Autodesk Inventor part; units mm, degrees
ref_plane "YZ Plane" through (0, 0, 0) normal (1, 0, 0) x (0, 1, 0)
ref_plane "XZ Plane" through (0, 0, 0) normal (0, 1, 0) x (-1, 0, 0)
ref_plane "XY Plane" through (0, 0, 0) normal (0, 0, 1) x (1, 0, 0)
sketch "Sketch2" plane through (0, 0, 0) normal (0, 0, 1) x (1, 0, 0)
  line L0 (0, 310) -> (0, 0)
  line L1 (0, 0) -> (10, 0)
  line L2 (10, 0) -> (10, 0)
  line L3 (10, 0) -> (80, 0)
  line L4 (80, 0) -> (80, 10)
  line L5 (80, 10) -> (10, 10)
  line L6 (10, 10) -> (10, 110)
  line L7 (10, 110) -> (80, 110)
  line L8 (80, 110) -> (80, 120)
  line L9 (80, 120) -> (10, 120)
  line L10 (10, 120) -> (10, 310)
  line L11 (10, 310) -> (0, 310)
  dimension "d12" = 100
  dimension "d13" = 10
  dimension "d14" = 10
  dimension "d15" = 10
  dimension "d16" = 10
  dimension "d17" = 190
  dimension "d18" = 310
  dimension "d19" = 80
extrude "Extrusion2" add sketch "Sketch2" along normal mid plane 10
properties part number "support" material "Steel"
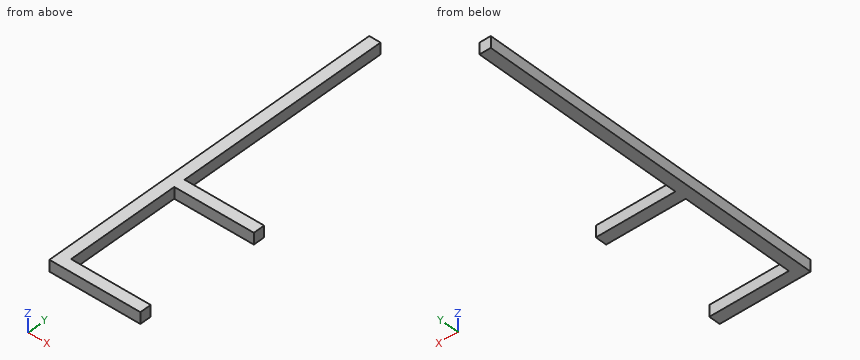
The model under review builds one solid part; all positions refer to its coordinate system, in mm. Round coordinates to 2 decimals unless told otherwise and drop trailing zeros. Write each loop counter-clockwise with the first axis right and the second up, starting at its lowest first coordinate (ties: lowest second). Pieces come first, ordered by that corner, then holes. Notation, with made-up numbers: (7, 15.25) - (12, 15.25) arc R20 cw to (12, 52.25) - close; hole circle Ø5 at (75, 33). An arc over 180 degrees is marked (long way). Use one line per item in the form item = value.
Q1. Consider section C-C (y = 149). State the section outline as (x, z) points.
Answer key:
outline = (0, -5) - (10, -5) - (10, 5) - (0, 5) - close
Q2. Consider section B-B (z = -2.25). State the section outline as (x, y) points, and give its area (3 significant figures).
Answer key:
outline = (0, 0) - (80, 0) - (80, 10) - (10, 10) - (10, 110) - (80, 110) - (80, 120) - (10, 120) - (10, 310) - (0, 310) - close
area = 4,500 mm2
Q3. For line 1 (Y direction, x = 19.5, z = 2.75); line 2 (X direction, y = 30, z = 2.5), list the stretches that pass through material, from the lowest coordinate up. Write a range as [from, to].
Answer key:
line_1 = [0, 10], [110, 120]
line_2 = [0, 10]
Q4. Consider section A-A (x = 50). State the section outline as (y, z) points.
Answer key:
outline = (0, -5) - (10, -5) - (10, 5) - (0, 5) - close; (110, -5) - (120, -5) - (120, 5) - (110, 5) - close
Q5. Insertion check: pin 1 Ø5 at (x, z) = (36.5, 0) entering from +Y; pin 2 Ø5 at (y, z) = (183.5, 1.5) entering from +X. Each pin has a flat end and moves straight along its axis. Give the tip position at first contact, or say it passes through.
Answer key:
pin_1 = 120
pin_2 = 10
